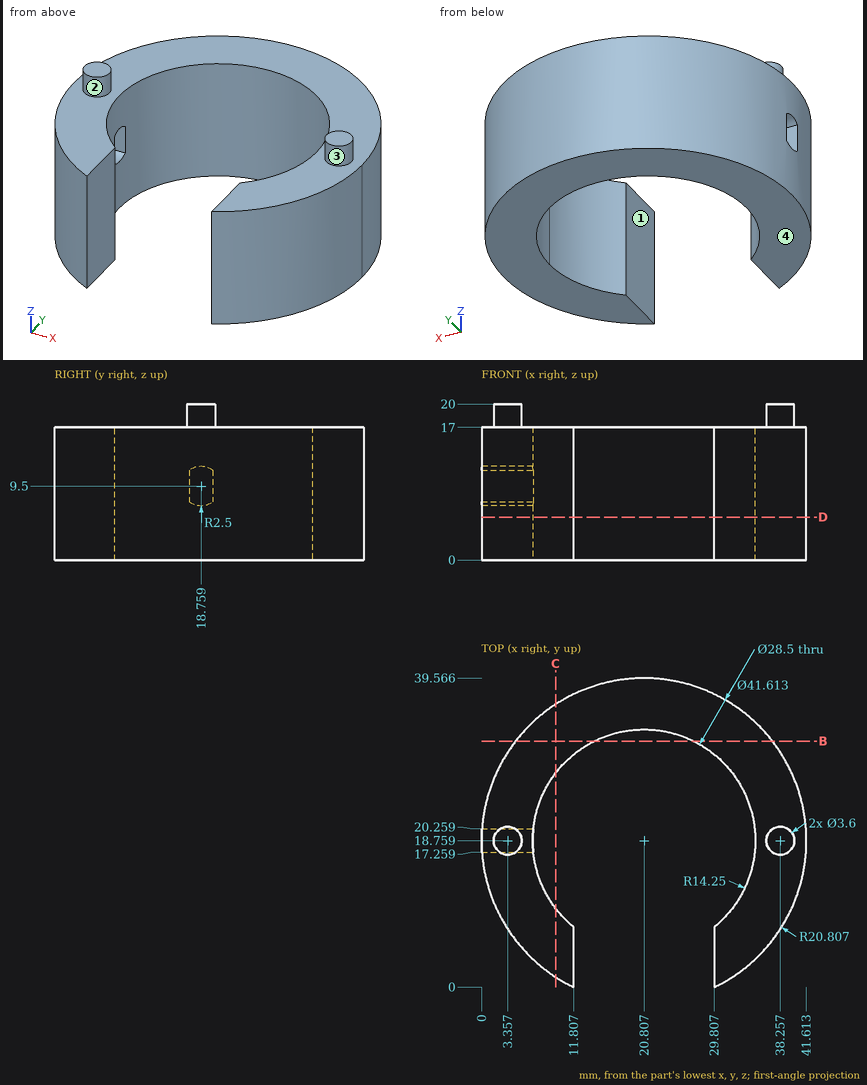
Could you check a few things on this drawing? It's one solid part, dimensions in mm from its lowest x, y, z. A direction names the side the tool comes from. Give positions to 0.01 mm unless a question says otherwise; leave off trailing zeros. Order: outer loops, then holes, each group sorted by start corner. A loop starts at its lowest first (then second) coordinate and runs counter-clockwise, first axis right, second up. Notation, with made-up numbers: M 40.25,-4 L 71.25,-4 A20 cw 71.25,16 Z; hole C -19.75,87 d4. An arc over 180 degrees is marked long. Use one line per item in the form item = value. Start each with the question number.
Item 1: If I drill on line 1 along Z through (x, y) = (31.5, 36); line 2 along X through (y, z) = (14.5, 6.75) (1 decimal); line 3 along X through (y, z) = (27, 4.75), over which ranges is the centre line in solid material (lowest first)?
Item 2: Will these pins go through, and if not, where does the flat tip stop? pin 1 Ø2 at (x, z) = (18.5, 16) entering from -Y; pin 2 Ø3 at (y, z) = (5.5, 14.5) entering from +X; pin 3 Ø2 at (x, y) = (29.5, 8) entering from +Z.
Item 3: We'd pull the mould along X, two halves only. Please class the marked faces 3 and 4: +X half, -X half, draft (parallel to the pull), parting line (faces both ways), or undercut.
Item 4: If we section it at C-C (x = 9.5): Write out the boundary of the cut face in (y, z) (1 decimal), then the cut area to 3 significant figures.
Item 5: For the marked faces 1 and 2, which set-ups out of +Z, -Z, +X, -X, +Y, -Y let a thin tool reach every point of the face, with its end or its side?
Item 6: If we section it at D-D (z = 5.5): Write out the boundary of the cut face in (x, y).
Item 7: If we section it at B-B (y = 31.5): Write out the boundary of the cut face in (x, z).
Outcome:
q1.line_1 = 0 to 17
q1.line_2 = 0.4 to 7.2, 34.4 to 41.2
q1.line_3 = 1.7 to 9.18, 32.43 to 39.91
q2.pin_1 = 32.62
q2.pin_2 = 37.97
q2.pin_3 = 17
q3.face_3 = undercut
q3.face_4 = draft
q4.outline = M 1.3,0 L 10.1,0 L 10.1,17 L 1.3,17 Z; M 27.4,0 L 36.2,0 L 36.2,17 L 27.4,17 Z
q4.area = 299 mm2
q5.face_1 = +Z, -Z, -Y
q5.face_2 = +Z
q6.outline = M 11.81,0 L 11.81,7.71 A14.25 cw long 29.81,7.71 L 29.81,0 A20.81 ccw long Z
q7.outline = M 4.36,0 L 14.42,0 L 14.42,17 L 4.36,17 Z; M 27.19,0 L 37.26,0 L 37.26,17 L 27.19,17 Z
